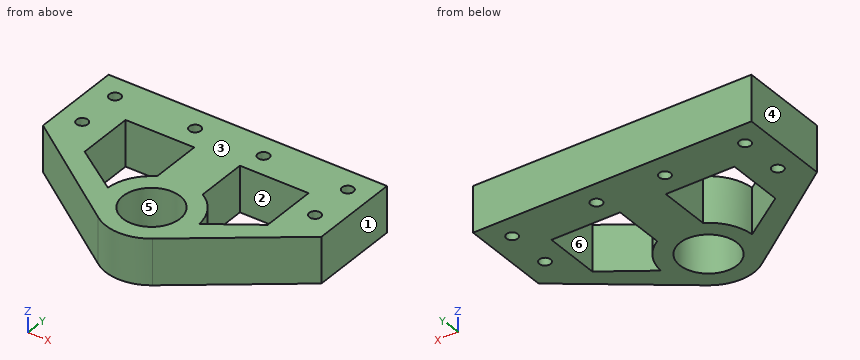
from build123d import *

# Parameters (mm, degrees)
SKETCH1_R           = 7.9375
BOSS_EXTRUDE1_DEPTH = 12.7
SKETCH2_R           = 1.5875
CUT_EXTRUDE1_DEPTH  = 12.7
CUT_EXTRUDE2_DEPTH  = 15.24
FILLET1_R           = 12.7


with BuildPart() as part:
    # Sketch1 → Boss-Extrude1 (new body)
    with BuildSketch(Plane.XY):
        Polygon((41.245841837, 19.276785714), (41.245841837, 44.676785714), (-36.224158163, 44.676785714), (-36.224158163, 19.276785714), (3.2200448, -9.183280125), align=None)
        with Locations((3.082341837, 6.576785714)):
            Circle(SKETCH1_R, mode=Mode.SUBTRACT)
    extrude(amount=BOSS_EXTRUDE1_DEPTH)

    # Sketch2 → Cut-Extrude1 (cut)
    with BuildSketch(Plane.XY.offset(12.7)):
        with Locations((-29.874158163, 38.326785714)):
            Circle(SKETCH2_R)
        with Locations((-29.874158163, 25.626785714)):
            Circle(SKETCH2_R)
        with Locations((34.895841837, 38.326785714)):
            Circle(SKETCH2_R)
        with Locations((34.895841837, 25.626785714)):
            Circle(SKETCH2_R)
        with Locations((-7.585658163, 38.326785714)):
            Circle(SKETCH2_R)
        with Locations((11.464341837, 38.326785714)):
            Circle(SKETCH2_R)
    extrude(amount=-CUT_EXTRUDE1_DEPTH, mode=Mode.SUBTRACT)

    # Sketch3 → Cut-Extrude2 (cut)
    with BuildSketch(Plane.XY.offset(12.7)):
        with BuildLine():
            Line((-22.381158163, 31.976785714), (-3.267658163, 31.976785714))
            Line((-3.267658163, 31.976785714), (-3.267658163, 17.575308342))
            ThreePointArc((-3.267658163, 17.575308342), (-7.722098193, 13.251669657), (-9.595109212, 7.333247809))
            Line((-9.595109212, 7.333247809), (-22.381158163, 16.12545158))
            Line((-22.381158163, 16.12545158), (-22.381158163, 31.976785714))
        make_face()
        with BuildLine():
            Line((9.432341837, 17.575308342), (9.432341837, 31.976785714))
            Line((9.432341837, 31.976785714), (28.545841837, 31.976785714))
            Line((28.545841837, 31.976785714), (28.545841837, 16.12545158))
            Line((28.545841837, 16.12545158), (15.754893995, 7.41130462))
            ThreePointArc((15.754893995, 7.41130462), (13.866177683, 13.284906497), (9.432341837, 17.575308342))
        make_face()
    extrude(amount=-CUT_EXTRUDE2_DEPTH, mode=Mode.SUBTRACT)

    # Fillet1
    fillet1_edges = [part.edges().sort_by_distance(p)[0] for p in [
        (3.2200448, -9.183280125, 6.35),
    ]]
    fillet(fillet1_edges, radius=FILLET1_R)


solid = part.part
Here's how the part is built. I have some questions about the finished solid (model axes, mm). Face numbers are marked on the shaded views. A direction names the side the tool comes from. Give positions to 0.01 mm unless a question says otherwise; leave off trailing zeros. Order: outer loops, then holes, each group sorted by start corner. A loop starts at its lowest first (then second) coordinate and runs counter-clockwise, first axis right, second up. Notation, with made-up numbers: (68.25, -19.5) -> (105.25, -19.5) arc R17 ccw to (105.25, 1.5) -> close; hole circle Ø4 at (29, -23.5). An arc over 180 degrees is marked (long way). Use a Markdown table: item, result. Add a question column.
Item 1: Imagine slicing it at A-A on y = 30.5. Please give me the cut outline in (x, z).
Item 2: Imagine slicing it at C-C on y = 11. Please give me the cut outline in (x, z).
Item 3: If we mould it in two halves opening along X, with no side actions, what happens to the marked faces 3, 4, 5 and 6? For each: pulls with the +X half, pulls with the -X half, needs draft (parallel to the pull), parting line crosses it, or undercut.
Item 4: I need wall thicknesses on line 1 (X direction, y = 27.5, z = 8.5); line 2 (Y direction, x = -7, z = 2.75); line 3 (X direction, y = 18, z = 2). Which ranges of each line are inside material? Lowest first, please.
Item 5: For the marked faces 1 and 2, which set-ups out of +Z, -Z, +X, -X, +Y, -Y let a thin tool reach every point of the face, with its end or its side?
Item 6: Imagine slicing it at D-D on z = 6.5. Give the number of separate pieces and of enclosed holes in the cut face, plus the area to 3 significant figures.
Item 7: Imagine slicing it at B-B on x = 17.5. Please give me the cut outline in (y, z), plus the area to 3 significant figures.
Item 8: Will these pins go through, and if not, where does the flat tip stop? pin 1 (6.5 mm diameter, centred on x = -10.5, z = 6, fed in from -Y); pin 2 (1.5 mm diameter, centred on y = 11, z = 10.5, fed in from -X); pin 3 (3 mm diameter, centred on x = 1, z = 10, fed in from -Y); pin 4 (3 mm diameter, centred on x = 11.46, y = 38.33, fed in from +Z).
Data:
| question | item | result |
|---|---|---|
| 1 | outline | (-36.22, 0) -> (-22.38, 0) -> (-22.38, 12.7) -> (-36.22, 12.7) -> close; (-3.27, 0) -> (9.43, 0) -> (9.43, 12.7) -> (-3.27, 12.7) -> close; (28.55, 0) -> (41.25, 0) -> (41.25, 12.7) -> (28.55, 12.7) -> close |
| 2 | outline | (-24.75, 0) -> (-14.93, 0) -> (-14.93, 12.7) -> (-24.75, 12.7) -> close; (-8.82, 0) -> (-3.51, 0) -> (-3.51, 12.7) -> (-8.82, 12.7) -> close; (9.67, 0) -> (14.99, 0) -> (14.99, 12.7) -> (9.67, 12.7) -> close; (21.02, 0) -> (30.19, 0) -> (30.19, 12.7) -> (21.02, 12.7) -> close |
| 3 | face 3 | needs draft |
| 3 | face 4 | pulls with the -X half |
| 3 | face 5 | undercut |
| 3 | face 6 | undercut |
| 4 | line 1 | x = -36.22 to -22.38, -3.27 to 9.43, 28.55 to 41.25 |
| 4 | line 2 | y = -1.81 to 14.3, 31.98 to 36.85, 39.8 to 44.68 |
| 4 | line 3 | x = -34.45 to -22.38, -3.27 to 9.43, 28.55 to 39.54 |
| 5 | face 1 | +Z, -Z, +X, +Y, -Y |
| 5 | face 2 | +Z, -Z |
| 6 | separate pieces | 1 |
| 6 | enclosed holes | 9 |
| 6 | area | 2,070 mm² |
| 7 | outline | (1.5, 0) -> (8.6, 0) -> (8.6, 12.7) -> (1.5, 12.7) -> close; (31.98, 0) -> (44.68, 0) -> (44.68, 12.7) -> (31.98, 12.7) -> close |
| 7 | area | 251 mm² |
| 8 | pin 1 | stops at y = -1.63 |
| 8 | pin 2 | stops at x = -25.79 |
| 8 | pin 3 | stops at y = -6.11 |
| 8 | pin 4 | passes through |
